Verification items for the finished model (mm, model axes). Face numbers are marked on the shaded views. Coordinates: 2 decimals unless noted, no trailing zeros. Order: outer loops, then holes, each group sorted by start corner. A loop starts at its lowest first (then second) coordinate and runs counter-clockwise, first axis right, second up.
Q1. Depth check by flat-ended pin: P1, Ø1.5, axis at y = 5, z = 4, coming from the -X side. Enter the tip coordinate at first touch or a pass-through.
Q2. Cross-section at A-A, the plane x = 0. Record the boundary of the cut face in (y, z).
Q3. Draft check along X on the marked faces 1, 2, 3 and 4. Enter one of: pulls with the +X half, pulls with the -X half, needs draft (parallel to the pull), parting line crosses it, or undercut.
Q4. Cross-section at C-C, the plane z = 0.95. Record the boundary of the cut face in (x, y).
Q5. Thickness scan on line 1 (Y direction, x = 0, z = 1.25); line 2 (X direction, y = -1.75, z = 3.45); line 3 (X direction, y = -4, z = 3.6). Record the ranges inside material, lowest first.
from build123d import *

# Parameters (mm, degrees)
ESBO_O1_R                                            = 8
RESSALTO_EXTRUS_O1_DEPTH                             = 5
FORMSENKUNG_F_R_M3_LINSENSENKSCHRAUBE_MI_D           = 3.2
FORMSENKUNG_F_R_M3_LINSENSENKSCHRAUBE_MI_DEPTH       = 20.87
FORMSENKUNG_F_R_M3_LINSENSENKSCHRAUBE_MI_CSINK_D     = 6.3
FORMSENKUNG_F_R_M3_LINSENSENKSCHRAUBE_MI_CSINK_ANGLE = 90
FORMSENKUNG_F_R_M3_LINSENSENKSCHRAUBE_MI_TIP         = 0.96137699
FILETE1_R                                            = 0.3


with BuildPart() as part:
    # Esboço1 → Ressalto-extrusão1 (new body)
    with BuildSketch(Plane.XY):
        Circle(ESBO_O1_R)
    extrude(amount=RESSALTO_EXTRUS_O1_DEPTH)

    # Formsenkung für M3 Linsensenkschraube mit Schlitz1
    with Locations(Plane.XY.offset(5)):
        with Locations((0, 0)):
            CounterSinkHole(FORMSENKUNG_F_R_M3_LINSENSENKSCHRAUBE_MI_D / 2, FORMSENKUNG_F_R_M3_LINSENSENKSCHRAUBE_MI_CSINK_D / 2, depth=FORMSENKUNG_F_R_M3_LINSENSENKSCHRAUBE_MI_DEPTH, counter_sink_angle=FORMSENKUNG_F_R_M3_LINSENSENKSCHRAUBE_MI_CSINK_ANGLE)
            with Locations((0, 0, -(FORMSENKUNG_F_R_M3_LINSENSENKSCHRAUBE_MI_DEPTH + FORMSENKUNG_F_R_M3_LINSENSENKSCHRAUBE_MI_TIP / 2))):  # 118° drill point
                Cone(0, FORMSENKUNG_F_R_M3_LINSENSENKSCHRAUBE_MI_D / 2, FORMSENKUNG_F_R_M3_LINSENSENKSCHRAUBE_MI_TIP, mode=Mode.SUBTRACT)

    # Filete1
    filete1_edges = [part.edges().sort_by_distance(p)[0] for p in [
        (-8, 0, 0),
    ]]
    fillet(filete1_edges, radius=FILETE1_R)


solid = part.part
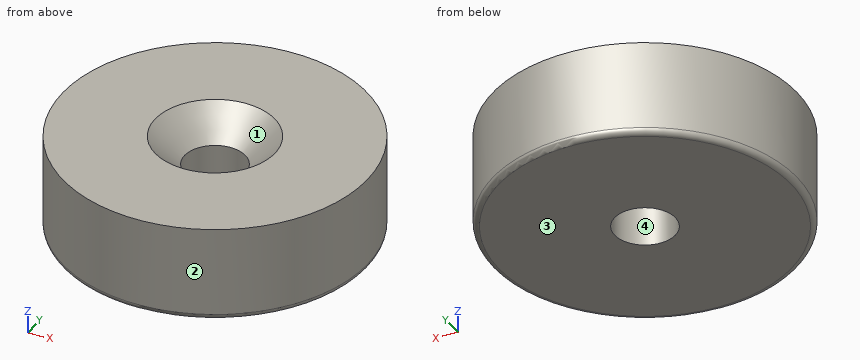
Check values:
1. P1: stops at x = -6.78
2. outline: (-8, 0.3) arc R0.3 ccw to (-7.7, 0) - (-1.6, 0) - (-1.6, 3.45) - (-3.15, 5) - (-8, 5) - close; (1.6, 0) - (7.7, 0) arc R0.3 ccw to (8, 0.3) - (8, 5) - (3.15, 5) - (1.6, 3.45) - close
3. face 1: undercut
3. face 2: parting line crosses it
3. face 3: needs draft
3. face 4: undercut
4. outline: circle Ø16 at (0, 0); hole circle Ø3.2 at (0, 0)
5. line 1: y = -8 to -1.6, 1.6 to 8
5. line 2: x = -7.81 to 7.81
5. line 3: x = -6.93 to 6.93
